Part model, mm, in its own coordinate system. A direction names the side the tool comes from. Give positions to 0.01 mm unless a question says otherwise; leave off trailing zeros. Order: outer loops, then holes, each group sorted by start corner. A loop starts at its lowest first (then second) coordinate and runs counter-clockwise, first axis right, second up. Notation, with made-up numbers: M 79.25,-18.5 L 96.25,-18.5 A36 ccw 96.25,16.5 Z; hole C 82,-28 d6. An arc over 180 degrees is marked long. One line per question, with ' | ' between items.
```python
from build123d import *

# Parameters (mm, degrees)
SKETCH1_W                          = 90
SKETCH1_H                          = 90
BOSS_EXTRUDE1_DEPTH                = 15
SKETCH2_R                          = 30
BOSS_EXTRUDE2_DEPTH                = 8.5
SKETCH3_R                          = 27
BOSS_EXTRUDE3_DEPTH                = 4
SKETCH4_R                          = 30
BOSS_EXTRUDE4_DEPTH                = 2.5
SKETCH5_R                          = 30
BOSS_EXTRUDE5_DEPTH                = 55.2
SKETCH6_R                          = 10
CUT_EXTRUDE1_DEPTH                 = 46
CUT_EXTRUDE1_DEPTH_BACK            = 46
SKETCH7_W                          = 20
SKETCH7_H                          = 64.311961004
CUT_EXTRUDE2_DEPTH                 = 55.2
SKETCH8_OUTSIDE_W                  = 124.398
SKETCH8_OUTSIDE_H                  = 124.398
SKETCH8_OUTSIDE_W_2                = 50
SKETCH8_OUTSIDE_H_2                = 73.670791152
CUT_EXTRUDE3_DEPTH                 = 60
CUT_EXTRUDE5_DEPTH                 = 21
CUT_EXTRUDE5_DEPTH_BACK            = 71
TAP_DRILL_FOR_M1_2X0_25_TAP1_D     = 48
TAP_DRILL_FOR_M1_2X0_25_TAP1_DEPTH = 25
TAP_DRILL_FOR_M1_2X0_25_TAP1_TIP   = 14.420654857
CIRPATTERN1_COUNT                  = 4
M16X1_5_TAPPED_HOLE1_D             = 14.5
M16X1_5_TAPPED_HOLE1_DEPTH         = 16
M16X1_5_TAPPED_HOLE1_TIP           = 4.356239488
SKETCH18_R                         = 1.7
CUT_EXTRUDE6_DEPTH                 = 46


with BuildPart() as part:
    # Sketch1 → Boss-Extrude1 (new body, symmetric)
    with BuildSketch(Plane(origin=(0, 0, 0), x_dir=(1, 0, 0), z_dir=(0, 1, 0))):
        Rectangle(SKETCH1_W, SKETCH1_H)
    extrude(amount=BOSS_EXTRUDE1_DEPTH, both=True)

    # Sketch2 → Boss-Extrude2 (add)
    with BuildSketch(Plane(origin=(0, 15, 0), x_dir=(1, 0, 0), z_dir=(0, 1, 0))):
        Circle(SKETCH2_R)
    extrude(amount=BOSS_EXTRUDE2_DEPTH)

    # Sketch3 → Boss-Extrude3 (add)
    with BuildSketch(Plane(origin=(0, 23.5, 0), x_dir=(1, 0, 0), z_dir=(0, 1, 0))):
        Circle(SKETCH3_R)
    extrude(amount=BOSS_EXTRUDE3_DEPTH)

    # Sketch4 → Boss-Extrude4 (add)
    with BuildSketch(Plane(origin=(0, 27.5, 0), x_dir=(1, 0, 0), z_dir=(0, 1, 0))):
        Circle(SKETCH4_R)
    extrude(amount=BOSS_EXTRUDE4_DEPTH)

    # Sketch5 → Boss-Extrude5 (add)
    with BuildSketch(Plane(origin=(0, -15, 0), x_dir=(-1, 0, 0), z_dir=(0, -1, 0))):
        Circle(SKETCH5_R)
    extrude(amount=BOSS_EXTRUDE5_DEPTH)

    # Sketch6 → Cut-Extrude1 (cut, two sides)
    with BuildSketch(Plane(origin=(0, 0, 0), x_dir=(0, 0, -1), z_dir=(1, 0, 0))) as cut_extrude1_sk:
        with Locations((0, -45)):
            Circle(SKETCH6_R)
    extrude(amount=CUT_EXTRUDE1_DEPTH, mode=Mode.SUBTRACT)
    extrude(cut_extrude1_sk.sketch, amount=-CUT_EXTRUDE1_DEPTH_BACK, mode=Mode.SUBTRACT)

    # Sketch7 → Cut-Extrude2 (cut)
    with BuildSketch(Plane(origin=(0, -70.2, 0), x_dir=(-1, 0, 0), z_dir=(0, -1, 0))):
        Rectangle(SKETCH7_W, SKETCH7_H)
    extrude(amount=-CUT_EXTRUDE2_DEPTH, mode=Mode.SUBTRACT)

    # Sketch8 outside → Cut-Extrude3 (cut)
    with BuildSketch(Plane(origin=(0, -15, 0), x_dir=(-1, 0, 0), z_dir=(0, -1, 0))):
        Rectangle(SKETCH8_OUTSIDE_W, SKETCH8_OUTSIDE_H)
        Rectangle(SKETCH8_OUTSIDE_W_2, SKETCH8_OUTSIDE_H_2, mode=Mode.SUBTRACT)
    extrude(amount=CUT_EXTRUDE3_DEPTH, mode=Mode.SUBTRACT)

    # Sketch10 → Cut-Extrude5 (cut, two sides)
    with BuildSketch(Plane(origin=(25, 0, 0), x_dir=(0, 0, -1), z_dir=(1, 0, 0))) as cut_extrude5_sk:
        with BuildLine():
            Line((28.284271247, -82.924550927), (-28.284271247, -82.924550927))
            Line((-28.284271247, -82.924550927), (-28.284271247, -50.2))
            ThreePointArc((-28.284271247, -50.2), (-17.320508076, -64.694897428), (0, -70.2))
            ThreePointArc((0, -70.2), (17.320508076, -64.694897428), (28.284271247, -50.2))
            Line((28.284271247, -50.2), (28.284271247, -82.924550927))
        make_face()
    extrude(amount=CUT_EXTRUDE5_DEPTH, mode=Mode.SUBTRACT)
    extrude(cut_extrude5_sk.sketch, amount=-CUT_EXTRUDE5_DEPTH_BACK, mode=Mode.SUBTRACT)

    # Tap Drill for M1.2x0.25 Tap1
    with Locations(Plane.ZX.offset(30)):
        with Locations((0, 0)):
            Hole(TAP_DRILL_FOR_M1_2X0_25_TAP1_D / 2, depth=TAP_DRILL_FOR_M1_2X0_25_TAP1_DEPTH)
            with Locations((0, 0, -(TAP_DRILL_FOR_M1_2X0_25_TAP1_DEPTH + TAP_DRILL_FOR_M1_2X0_25_TAP1_TIP / 2))):  # 118° drill point
                Cone(0, TAP_DRILL_FOR_M1_2X0_25_TAP1_D / 2, TAP_DRILL_FOR_M1_2X0_25_TAP1_TIP, mode=Mode.SUBTRACT)

    # Sketch15 → M12 Tapped Hole1 (revolve, cut)
    with BuildSketch(Plane(origin=(31.819805153, 15, -31.819805153), x_dir=(0, 0, 1), z_dir=(1, 0, 0))):
        Polygon((0, 0), (0, 23.064389157), (5.1, 20), (5.1, 0), align=None)
    m12_tapped_hole1 = revolve(axis=Axis((31.819805153, 21.35, -31.819805153), (0, -1, 0)), mode=Mode.SUBTRACT)

    # CirPattern1: M12 Tapped Hole1 ×4 about axis
    cirpattern1_axis = Axis((0, 0, 0), (0, 1, 0))
    for i in range(1, CIRPATTERN1_COUNT):
        add(m12_tapped_hole1.rotate(cirpattern1_axis, i * 360 / CIRPATTERN1_COUNT), mode=Mode.SUBTRACT)

    # M16x1.5 Tapped Hole1
    with Locations(Plane(origin=(0, 0, -45), x_dir=(-1, 0, 0), z_dir=(0, 0, -1))):
        with Locations((0, 0)):
            Hole(M16X1_5_TAPPED_HOLE1_D / 2, depth=M16X1_5_TAPPED_HOLE1_DEPTH)
            with Locations((0, 0, -(M16X1_5_TAPPED_HOLE1_DEPTH + M16X1_5_TAPPED_HOLE1_TIP / 2))):  # 118° drill point
                Cone(0, M16X1_5_TAPPED_HOLE1_D / 2, M16X1_5_TAPPED_HOLE1_TIP, mode=Mode.SUBTRACT)

    # Sketch18 → Cut-Extrude6 (cut)
    with BuildSketch(Plane(origin=(0, 0, -45), x_dir=(-1, 0, 0), z_dir=(0, 0, -1))):
        Circle(SKETCH18_R)
    extrude(amount=-CUT_EXTRUDE6_DEPTH, mode=Mode.SUBTRACT)


solid = part.part
```
1. Slice it at C-C on z = 39. Give the cut face in (x, y).
Worked out:
outline: M -45,-15 L 45,-15 L 45,15 L -45,15 Z
2. Slice it at A-A on y = -30. Give the cut face in (x, z), then the cut area to 3 significant figures.
Worked out:
outline: M -25,-16.58 A30 ccw -10,-28.28 L -10,28.28 A30 ccw -25,16.58 Z; M 10,-28.28 A30 ccw 25,-16.58 L 25,16.58 A30 ccw 10,28.28 Z | area: 1,420 mm2
3. Slice it at B-B on y = -45. Give the cut face in (x, z), then the cut area to 3 significant figures.
Worked out:
outline: M -25,-16.58 A30 ccw -10,-28.28 L -10,-10 L -25,-10 Z; M -25,10 L -10,10 L -10,28.28 A30 ccw -25,16.58 Z; M 10,-28.28 A30 ccw 25,-16.58 L 25,-10 L 10,-10 Z; M 10,10 L 25,10 L 25,16.58 A30 ccw 10,28.28 Z | area: 825 mm2
4. Tool access for faces 4 (the flat face through (-25, -36, -7)), 5 (the cylindrical face through (3.35, -6.43, -36.89)), 6 (the cylindrical face through (-18.56, -34.17, -23.57)), 7 (the flat face through (-1, 15, -31)), 8 (the cylindrical face through (18, -34, -24)): list every direction of +Z, -Z, +X, -X, +Y, -Y with a clear straight run to the whole face (end or side of a thin tool).
Worked out:
face 4: +Z, -Z, -X, -Y | face 5: -Z | face 6: -Z, -X, -Y | face 7: +Y | face 8: -Z, +X, -Y
5. Probe L1, parallel to Y at x = -29, z = -1.5; L2, parallel to X at y = -19, z = 10.5; L3, parallel to X at y = 14, z = -31. List the from-to ranges inside material, lowest first. Write a range as from..to.
Worked out:
L1: y = -15..23.5, 27.5..30 | L2: x = -25..-10, 10..25 | L3: x = -45..-36.85, -26.79..26.79, 36.85..45
6. Mould opens along Z. For faces 1 (the flat face through (45, 0, 1)), 2 (the conical face through (0.444, -1.999, -25.874)), 3 (the conical face through (31.07, -7.53, -31.34)) say: released by +Z, released by -Z, zero draft, split by the parting line, or undercut.
Worked out:
face 1: zero draft | face 2: released by -Z | face 3: undercut
7. Slice it at D-D on y = 21.5. Give the cut face in (x, z).
Worked out:
outline: C 0,0 d60; hole C 0,0 d48
8. Drop flat-ended pins along their axis: pin 1 (8 mm diameter, centred on x = -31.82, z = 31.82, fed in from -Y); pin 2 (16.5 mm diameter, centred on x = 0, y = 0, fed in from -Z); pin 3 (5 mm diameter, centred on x = 33.5, z = -7, fed in from +Y); pin 4 (18 mm diameter, centred on x = 8.5, z = -10.5, fed in from +Y). Give the stop position or say it passes through.
Worked out:
pin 1: stops at y = -15 | pin 2: stops at z = -45 | pin 3: stops at y = 15 | pin 4: stops at y = 4.1
